```python
from build123d import *

# Parameters (mm, degrees)
ESQUISSE1_R             = 10
BOSS_EXTRU_1_DEPTH      = 10
ESQUISSE2_R             = 5
BOSS_EXTRU_2_DEPTH      = 6
ESQUISSE3_R             = 2.5
ENL_V_MAT_EXTRU_1_DEPTH = 22.354156504
ESQUISSE4_W             = 8
ESQUISSE4_H             = 5


with BuildPart() as part:
    # Esquisse1 → Boss.-Extru.1 (new body)
    with BuildSketch(Plane.XY):
        Circle(ESQUISSE1_R)
    extrude(amount=BOSS_EXTRU_1_DEPTH)

    # Esquisse2 → Boss.-Extru.2 (add)
    with BuildSketch(Plane.XY.offset(10)):
        Circle(ESQUISSE2_R)
    extrude(amount=BOSS_EXTRU_2_DEPTH)

    # Esquisse3 → Enlèv. mat.-Extru.1 (cut, through all)
    with BuildSketch(Plane.XY.offset(16)):
        Circle(ESQUISSE3_R)
    extrude(amount=-ENL_V_MAT_EXTRU_1_DEPTH, mode=Mode.SUBTRACT)

    # Esquisse4 → Enlèvement de matière-Révolution1 (revolve, cut)
    with BuildSketch(Plane(origin=(0, 0, 0), x_dir=(0, 0, -1), z_dir=(1, 0, 0)), mode=Mode.PRIVATE) as enl_vement_de_mati_re_r_volution1_sk:
        with Locations((-5, 7.5)):
            Rectangle(ESQUISSE4_W, ESQUISSE4_H)
    revolve(enl_vement_de_mati_re_r_volution1_sk.sketch.rotate(Axis((0, 0, 0), (0, 0, 1)), 90), axis=Axis((0, 0, 0), (0, 0, 1)), mode=Mode.SUBTRACT)


solid = part.part
```
For this review, take the finished solid that the model builds, in its own axes (mm). A direction names the side the tool comes from. Give positions to 0.01 mm unless a question says otherwise; leave off trailing zeros. Loops run counter-clockwise (first coordinate to the right, second up) from the corner with the lowest first, then second, coordinate; pieces in that order, holes last. Notation, with made-up numbers: M 41,50.25 L 99,50.25 A27 ccw 99,87.25 Z; hole C -22,79 d4. An arc over 180 degrees is marked long. One line per item, written item: value. Start each with the question number.
Q1. Add section D-D (x = -6). Give the boundary of the cut face in (y, z), and give its area (3 significant figures).
Q2. Clearance check with flat-ended pins moving along their axes: pin 1 Ø1.5 at (y, z) = (-7, 1.5) entering from +X; pin 2 Ø2 at (x, y) = (-6.5, -4) entering from +Z; pin 3 Ø1.5 at (y, z) = (2, 3.5) entering from +X; pin 4 Ø2 at (x, z) = (-8, 2.5) entering from +Y. State where each tip first meets the part, or that it passes through.
Q3. Add section A-A (x = 0). Give the boundary of the cut face in (y, z), and give its area (3 significant figures).
Q4. Machinability: for faces 1 (the face through (-1.08, -4.88, 12.96)), 2 (the face through (-2.17, -9.76, 9.49)), 3 (the face through (2, -5, 9)), which of the approach directions +Z, -Z, +X, -X, +Y, -Y give a long, thin tool a straight path to every point of the face, cutting with its end or side? Answer none if there is none.
Q5. Draft analysis for pull direction Z (two halves, no side actions). For faces 4 (the face through (2, -2, 0)), 5 (the face through (2, -5, 1)), 6 (the face through (-5, -2, 10)), state which applies: released by +Z, released by -Z, zero draft, split by the parting line, or undercut.
Q6. Add section B-B (y = 8). Give the boundary of the cut face in (x, z), and give its area (3 significant figures).
Q7. Add section C-C (z = 8.25). Give the boundary of the cut face in (x, y).
Q8. For L1, parallel to Y at x = 0, z = 6.75; L2, parallel to Z at x = -8, y = 5.5; L3, parallel to Y at x = -1.5, z = 2, list the stretches that pass through material, from the lowest coordinate up.
Reply:
1. outline: M -8,0 L 8,0 L 8,1 L -8,1 Z; M -8,9 L 8,9 L 8,10 L -8,10 Z
1. area: 32.0 mm²
2. pin 1: x = 7.65
2. pin 2: z = 10
2. pin 3: x = 4.84
2. pin 4: through
3. outline: M -10,0 L -2.5,0 L -2.5,16 L -5,16 L -5,10 L -10,10 L -10,9 L -5,9 L -5,1 L -10,1 Z; M 2.5,0 L 10,0 L 10,1 L 5,1 L 5,9 L 10,9 L 10,10 L 5,10 L 5,16 L 2.5,16 Z
3. area: 100 mm²
4. face 1: +Z
4. face 2: +Z, -Z
4. face 3: none
5. face 4: released by -Z
5. face 5: undercut
5. face 6: released by +Z
6. outline: M -6,0 L 6,0 L 6,1 L -6,1 Z; M -6,9 L 6,9 L 6,10 L -6,10 Z
6. area: 24.0 mm²
7. outline: C 0,0 d10; hole C 0,0 d5
8. L1: -5 to -2.5, 2.5 to 5
8. L2: 0 to 1, 9 to 10
8. L3: -4.77 to -2, 2 to 4.77
